```python
from build123d import *

# Parameters (mm, degrees)
EXTRUDE_1_DEPTH     = 900
CUT_EXTRUDE_1_DEPTH = 4
CUT_EXTRUDE_2_DEPTH = 4


with BuildPart() as part:
    # Эскиз1 → Вытянуть-Тонкостенный1 (new body)
    with BuildSketch(Plane(origin=(0, 0, 0), x_dir=(1, 0, 0), z_dir=(0, 1, 0))):
        Polygon((0, 50), (0, 0), (50, 0), (50, 4), (4, 4), (4, 50), align=None)
    extrude(amount=EXTRUDE_1_DEPTH)

    # Эскиз3 → Вырез-Вытянуть1 (cut)
    with BuildSketch(Plane.XY):
        Polygon((0, 900), (50, 900), (0, 886.602540378), align=None)
    extrude(amount=-CUT_EXTRUDE_1_DEPTH, mode=Mode.SUBTRACT)

    # Эскиз4 → Вырез-Вытянуть2 (cut)
    with BuildSketch(Plane.ZY):
        Polygon((0, 900), (-50, 900), (-50, 887), (0, 886.602540378), align=None)
    extrude(amount=-CUT_EXTRUDE_2_DEPTH, mode=Mode.SUBTRACT)


solid = part.part
```
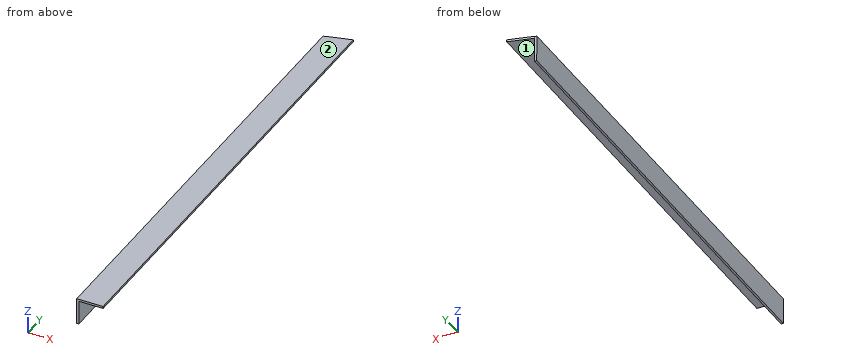
Here's how the part is built. I have some questions about the finished solid (model axes, mm). Face numbers are marked on the shaded views. A direction names the side the tool comes from. Coordinates: 2 decimals unless noted, no trailing zeros. Order: outer loops, then holes, each group sorted by start corner. A loop starts at its lowest first (then second) coordinate and runs counter-clockwise, first axis right, second up. Notation, with made-up numbers: M 89,-5 L 117,-5 A11 ccw 117,2 Z; hole C 88,11.25 d10. An arc over 180 degrees is marked long. Answer as a JSON object with one key per item and string values. Group by question number.
(1) Suppose I cut it at C-C, the plane z = -32.5. Please give me the cut outline in (x, y).
(2) For pin 1 (4 mm diameter, centred on y = 711, z = -42, fed in from -X); pin 2 (1.5 mm diameter, centred on x = 7, y = 327, fed in from -Z); pin 3 (5 mm diameter, centred on y = 753.5, z = -17.5, fed in from +X); pin 4 (1.2 mm diameter, centred on y = 887.5, z = -2.5, fed in from -X), each with a flat end and sliding along its axis, tell me the tip position at first contact or that it passes through.
(3) Suppose I cut it at A-A, the plane y = 670. Please give me the cut outline in (x, z), then the cut area to 3 significant figures.
(4) Suppose I cut it at B-B, the plane x = 35. Please give me the cut outline in (y, z).
(5) I need wall thicknesses on probe 1 along Z at (x, y) = (47, 612.5); probe 2 along X at (y, z) = (116, -27); probe 3 along Y at (x, z) = (2, -28.5). Which ranges of each line are inside material? Lowest first, please.
(6) Which directions (+Z, -Z, +X, -X, +Y, -Y) give clear straight access to the entire face, cutting with the end or side of a thin tool? Please do the marked faces 1 and 2.
Values found:
{
 "1": {"outline": "M 0,0 L 4,0 L 4,886.86 L 0,886.86 Z"},
 "2": {"pin 1": "stops at x = 0", "pin 2": "stops at z = -4", "pin 3": "stops at x = 4", "pin 4": "stops at x = 4"},
 "3": {"outline": "M 0,-50 L 4,-50 L 4,-4 L 50,-4 L 50,0 L 0,0 Z", "area": "384 mm^2"},
 "4": {"outline": "M 0,-4 L 895.98,-4 L 895.98,0 L 0,0 Z"},
 "5": {"probe 1": "z = -4 to 0", "probe 2": "x = 0 to 4", "probe 3": "y = 0 to 886.83"},
 "6": {"face 1": "-Z, +X, +Y, -Y", "face 2": "+Z, +X, -X, +Y, -Y"}
}
